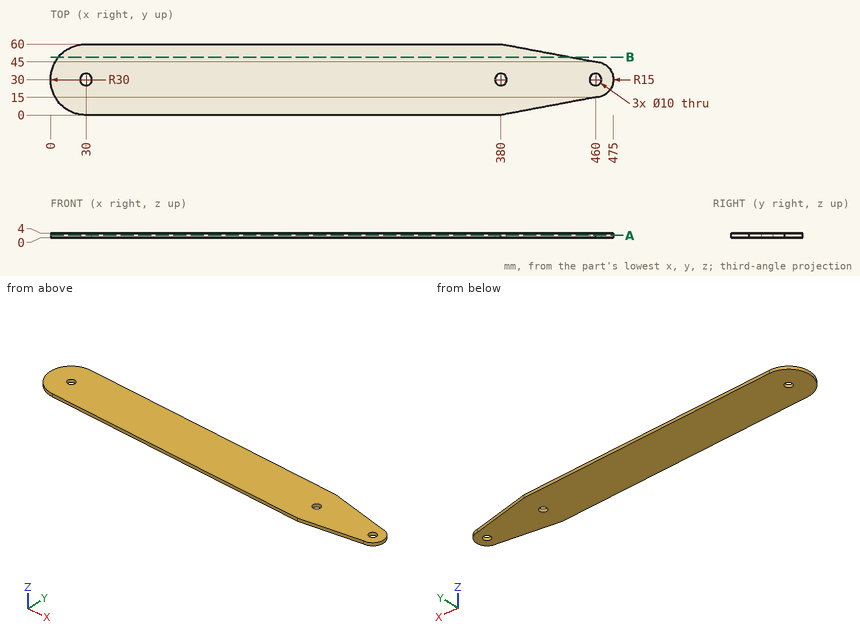
Can you work these out from the drawing? Everything is in mm from the part's minimum corner. Give positions to 0.01 mm unless a question says otherwise; leave off trailing zeros. Order: outer loops, then holes, each group sorted by start corner. A loop starts at its lowest first (then second) coordinate and runs counter-clockwise, first axis right, second up. Notation, with made-up numbers: M 58,7 L 91,7 A18 cw 91,23 Z; hole C 51.25,-24.5 d9. An arc over 180 degrees is marked long. One line per question, with ' | ' between items.
1. I want a section at B-B (y = 49). List the corners of the cut face in (x, z) for me, and give its area (3 significant figures).
Results:
outline: M 6.78,0 L 438.67,0 L 438.67,4 L 6.78,4 Z | area: 1,730 mm²
2. If I drill on line 1 (Y direction, x = 380, z = 1.45); line 2 (Y direction, x = 460, z = 1.65); line 3 (X direction, y = 37, z = 2.95), over which ranges is the centre line in solid material (lowest first)?
Results:
line 1: 0 to 25, 35 to 60 | line 2: 15 to 25, 35 to 45 | line 3: 0.83 to 473.27
3. I want a section at A-A (z = 2.05). List the corners of the cut face in (x, y) for me.
Results:
outline: M 30,0 L 380,0 L 460,15 A15 ccw 460,45 L 380,60 L 30,60 A30 ccw Z; hole C 30,30 d10; hole C 380,30 d10; hole C 460,30 d10
4. I'm going to push flat-ended pins straight in: pin 1 (1 mm diameter, centred on y = 25.5, z = 3, fed in from -X); pin 2 (1 mm diameter, centred on y = 34.5, z = 1.5, fed in from +X); pin 3 (9 mm diameter, centred on x = 30, y = 30, fed in from -Z); pin 4 (2 mm diameter, centred on y = 53.5, z = 1.5, fed in from -X). Where does each tip first touch, or does it pass through?
Results:
pin 1: x = 0.27 | pin 2: x = 474.46 | pin 3: through | pin 4: x = 10.16
